Input: part model. Units: mm. Frame: model coordinates. Give positions to 0.01 mm unless a question says otherwise; leave off trailing zeros. Loops run counter-clockwise (first coordinate to the right, second up) from the corner with the lowest first, then second, coordinate; pieces in that order, holes last. Notation, with made-up numbers: (22, 45.25) - (78, 45.25) arc R16 ccw to (78, 66.25) - close; hole circle Ø7 at (-13, 84.5). An arc over 180 degrees is marked (long way). One line per item, written item: value.
from build123d import *

# Parameters (mm, degrees)
SKETCH4_R           = 11.5
SKETCH4_R_2         = 1.5
BOSS_EXTRUDE1_DEPTH = 5


with BuildPart() as part:
    # Sketch4 → Boss-Extrude1 (new body)
    with BuildSketch(Plane.XY):
        with BuildLine():
            Line((-10.087403903, 107.088819702), (9.912596097, 107.088819702))
            ThreePointArc((9.912596097, 107.088819702), (20.519197815, 102.695421419), (24.912596097, 92.088819702))
            Line((24.912596097, 92.088819702), (24.912596097, 7.088819702))
            Line((24.912596097, 7.088819702), (-25.087403903, 7.088819702))
            Line((-25.087403903, 7.088819702), (-25.087403903, 92.088819702))
            ThreePointArc((-25.087403903, 92.088819702), (-20.694005621, 102.695421419), (-10.087403903, 107.088819702))
        make_face()
        with Locations((-0.087403903, 82.088819702)):
            Circle(SKETCH4_R, mode=Mode.SUBTRACT)
        with Locations((15.412596097, 66.588819702)):
            Circle(SKETCH4_R_2, mode=Mode.SUBTRACT)
        with Locations(Location((-15.587403903, 66.588819702, 0), (0, 0, 180))):
            Circle(SKETCH4_R_2, mode=Mode.SUBTRACT)
        with Locations(Location((15.412596097, 97.588819702, 0), (0, 0, 180))):
            Circle(SKETCH4_R_2, mode=Mode.SUBTRACT)
        with Locations((-15.587403903, 97.588819702)):
            Circle(SKETCH4_R_2, mode=Mode.SUBTRACT)
        with Locations((-8.087403903, 42.088819702)):
            Circle(SKETCH4_R_2, mode=Mode.SUBTRACT)
        with Locations(Location((7.912596097, 42.088819702, 0), (0, 0, 180))):
            Circle(SKETCH4_R_2, mode=Mode.SUBTRACT)
    extrude(amount=BOSS_EXTRUDE1_DEPTH)


solid = part.part
Item 1: Section C-C, the plane z = 2.8. Output: boundary loops of the cut face in (x, y), and give its area (3 significant figures).
Verdict:
outline: (-25.09, 7.09) - (24.91, 7.09) - (24.91, 92.09) arc R15 ccw to (9.91, 107.09) - (-10.09, 107.09) arc R15 ccw to (-25.09, 92.09) - close; hole circle Ø3 at (-15.59, 66.59); hole circle Ø3 at (-15.59, 97.59); hole circle Ø23 at (-0.09, 82.09); hole circle Ø3 at (-8.09, 42.09); hole circle Ø3 at (7.91, 42.09); hole circle Ø3 at (15.41, 66.59); hole circle Ø3 at (15.41, 97.59)
area: 4,450 mm^2
Item 2: Material intervals for L1, parallel to Y at x = -15.5, z = 1.65; L2, parallel to X at y = 97.5, z = 0.45; L3, parallel to Y at x = -0.5, z = 2.1, sorted ascending.
Verdict:
L1: y = 7.09 to 65.09, 68.09 to 96.09, 99.09 to 106.08
L2: x = -24.08 to -17.08, -14.09 to 13.92, 16.91 to 23.9
L3: y = 7.09 to 70.6, 93.58 to 107.09
Item 3: Section A-A, the plane x = 4. Output: boundary loops of the cut face in (y, z).
Verdict:
outline: (7.09, 0) - (71.34, 0) - (71.34, 5) - (7.09, 5) - close; (92.84, 0) - (107.09, 0) - (107.09, 5) - (92.84, 5) - close
Item 4: Section D-D, the plane x = 21. Output: boundary loops of the cut face in (y, z), and give its area (3 significant figures).
Verdict:
outline: (7.09, 0) - (102.19, 0) - (102.19, 5) - (7.09, 5) - close
area: 476 mm^2
Item 5: Pin query (flat end, axial travel): P1, Ø2.5, axis at x = 15.41, y = 97.59, coming from the +Z side. Return the tip coordinate at first contact, or that it passes through.
Verdict:
P1: passes through
Item 6: Section B-B, the plane y = 72. Output: boundary loops of the cut face in (x, z), and give its area (3 significant figures).
Verdict:
outline: (-25.09, 0) - (-5.61, 0) - (-5.61, 5) - (-25.09, 5) - close; (5.43, 0) - (24.91, 0) - (24.91, 5) - (5.43, 5) - close
area: 195 mm^2
Item 7: Draft query along Y for faces 1 (the face through (-8.283, 43.576, 2.465)), 2 (the face through (-20.81, 102.58, 2.46)), 3 (the face through (24.913, 50, 2)). Return one class per face: pulls with the +Y half, pulls with the -Y half, needs draft (parallel to the pull), parting line crosses it, or undercut.
Verdict:
face 1: undercut
face 2: pulls with the +Y half
face 3: needs draft
